Autodesk Inventor part; units mm, degrees
ref_plane "YZ Plane" through (0, 0, 0) normal (1, 0, 0) x (0, 1, 0)
ref_plane "XZ Plane" through (0, 0, 0) normal (0, 1, 0) x (-1, 0, 0)
ref_plane "XY Plane" through (0, 0, 0) normal (0, 0, 1) x (1, 0, 0)
sketch "Skizze5" plane through (0, 0, 0) normal (1, 0, 0) x (0, 1, 0)
  line L0 (0, 0) -> (0, 0)
  line L1 (0, 0) -> (4.4737, 0.486)
  line L2 (4.4737, 0.486) -> (10.9319, -0.2498)
  line L3 (10.9319, -0.2498) -> (10.9319, -0.2498)
  line L4 (10.9319, -0.2498) -> (10.9319, 5.2858)
  line L5 (10.9319, 5.2858) -> (4.4737, 6.0216)
  line L6 (0, 3.5206) -> (0, 0)
  line L7 (0, 3.5206) -> (4.4737, 4.0066)
  line L8 (4.4737, 8.0188) -> (4.4737, 2.9641) construction
  line L9 (4.4737, 6.0216) -> (4.4737, 4.0066)
  dimension "d21" = 0
  dimension "d22" = 6.2
  dimension "d23" = 6.5
  dimension "d24" = 4.5
  dimension "d25" = 6.5
  dimension "d26" = 5.5
  dimension "d27" = 3.5
extrude "Extrusion3" add sketch "Skizze5" along normal blind 8
sketch "Skizze6" plane through (8, 10.9319, -0.2498) normal (0, -0.1132, -0.9936) x (-1, 0, 0)
  circle A0 centre (4, -3.25) radius 2.425
  line L0 (4, 0.2781) -> (4, -10.3498)
  line L1 (-1.6335, -3.25) -> (9.1615, -3.25)
  line L2 (8, -6.5) -> (8, 0)
  line L3 (8, 0) -> (0, 0)
  point P0 (8, -10.8899)
  point P1 (8, -1.2477)
  point P2 (4, -0.9743)
  point P3 (8, -3.25)
  point P4 (4, 0)
  dimension "d30" = 4.85
extrude "Extrusion4" cut sketch "Skizze6" against normal through all contours L1 L0 A0 | A0 L0 L1 | L0 L1 A0 | A0 L1 L0
sketch "Skizze7" plane through (8, 4.4737, 0.486) normal (0, 0.108, -0.9942) x (-1, 0, 0)
  line L0 (-0.5646, -2.25) -> (9.8389, -2.25)
  line L1 (4, -0.832) -> (4, -8.1647)
  circle A0 centre (4, -2.25) radius 1.65
  line L2 (8, -4.5) -> (8, 0)
  line L3 (8, -4.5) -> (0, -4.5)
  point P0 (4, -5.6763)
  point P1 (8, -2.25)
  point P2 (8, -2.25)
  point P3 (4, -4.5)
  dimension "d33" = 3.3
extrude "Extrusion5" cut sketch "Skizze7" against normal through all contours A0 L0 | L0 L1 A0 | L0 A0 L1
chamfer "Fase2" distance 0.5 angle 45 4 edges at (8, 10.9319, 2.518) (0, 10.9319, 2.518) (8, 4.4737, 5.0141) (0, 4.4737, 5.0141)
ref_plane "Arbeitsebene3" through (0, 10.9319, -0.2498) normal (0, 0, 1) x (1, 0, 0)
sketch "Skizze11" plane through (0, 10.9319, -0.2498) normal (0, 0, 1) x (1, 0, 0)
  line L0 (0.5, 0) -> (7.5, 0)
  line L1 (8, -0.5) -> (7.5, 0)
  line L2 (8, -6.4582) -> (8, -0.5)
  line L3 (8, -10.9319) -> (8, -6.4582)
  line L4 (0, -10.9319) -> (8, -10.9319)
  line L5 (0, -10.9319) -> (0, -6.4582)
  line L6 (0, -6.4582) -> (0, -0.5)
  line L7 (0.5, 0) -> (0, -0.5)
extrude "Extrusion9" add sketch "Skizze11" along normal blind 1
sketch "Skizze12" plane through (0.5, 4.4737, 6.0216) normal (0, 0.1132, 0.9936) x (1, 0, 0)
  circle A0 centre (3.5, 3.8766) radius 2.425
  point P0 (-0.5, -3.7633)
extrude "Extrusion10" cut sketch "Skizze12" against normal through all
sketch "Skizze13" plane through (0, 0, 3.5206) normal (0, -0.108, 0.9942) x (1, 0, 0)
  circle A0 centre (4, 1.8698) radius 1.65
  point P0 (0, -0.3802)
extrude "Extrusion11" cut sketch "Skizze13" against normal through all
chamfer "Fase4" distance 0.5 angle 45 3 edges at (8, 5.2159, -0.2498) (4, 10.9319, -0.2498) (0, 5.2159, -0.2498)
chamfer "Fase5" distance 1.5 angle 45 2 edges at (8, 0, 1.8854) (0, 0, 1.8854)
properties part number "led_holder_v13"
Input: part model. Units: mm. Frame: model coordinates. A direction names the side the tool comes from. Coordinates: 2 decimals unless noted, no trailing zeros. Order: outer loops, then holes, each group sorted by start corner. A loop starts at its lowest first (then second) coordinate and runs counter-clockwise, first axis right, second up. Notation, with made-up numbers: M -11.5,74.25 L 39.5,74.25 A16 cw 39.5,97.25 Z; hole C 36.25,69.5 d5. An arc over 180 degrees is marked long. Answer in a Markdown table with one row per item.
(1) Material intervals for line 1 (Y direction, x = 3.5, z = 0.75); line 2 (Y direction, x = 3.75, z = 3); line 3 (Y direction, x = 1.25, z = 1.5), sorted ascending. Write a range as [from, to].
Numbers:
| item | result |
|---|---|
| line 1 | y = [0, 0.6], [3.76, 5.39], [10.16, 10.93] |
| line 2 | y = [0, 0.3], [3.58, 5.6], [10.46, 10.93] |
| line 3 | y = [0.25, 10.93] |
(2) Section query B-B, the plane x = 6.25. Output: boundary loops of the cut face in (y, z), plus the area to 3 significant figures.
Numbers:
| item | result |
|---|---|
| outline | M 0,-0.25 L 6.75,-0.25 L 7.43,5.69 L 4.47,6.02 L 4.47,4.01 L 0,3.52 Z; M 8.57,-0.25 L 10.43,-0.25 L 10.93,0.25 L 10.93,5.29 L 9.22,5.48 Z |
| area | 45.3 mm^2 |
(3) Contact query for flat-ended pins moving along their axis: pin 1 Ø0.6 at (x, z) = (2.5, 4.5) entering from -Y; pin 2 Ø4 at (x, y) = (5, 6.5) entering from -Z. Output: stop coordinate, or through.
Numbers:
| item | result |
|---|---|
| pin 1 | stops at y = 4.47 |
| pin 2 | stops at z = -0.25 |
(4) Section query D-D, the plane z = 1. Give the number of separate pieces and of enclosed holes in the cut face, plus the area to 3 significant figures.
Numbers:
| item | result |
|---|---|
| separate pieces | 1 |
| enclosed holes | 2 |
| area | 57.8 mm^2 |
(5) Access query for faces 1 (the flat face through (4, 0, 2)), 2 (the flat face through (4, 4.474, 5)). Directions: +Z, -Z, +X, -X, +Y, -Y. A direction counts if a zero-diameter tool reaches every point of the face in a straight line with its end or side. Return the directions, or none.
Numbers:
| item | result |
|---|---|
| face 1 | +Z, -Z, +X, -X, -Y |
| face 2 | +Z, +X, -X, -Y |
(6) Section query C-C, the plane x = 1. Output: boundary loops of the cut face in (y, z), plus the area to 3 significant figures.
Numbers:
| item | result |
|---|---|
| outline | M 0.5,-0.25 L 10.43,-0.25 L 10.93,0.25 L 10.93,5.29 L 4.47,6.02 L 4.47,4.01 L 0.5,3.57 Z |
| area | 54.1 mm^2 |
(7) Section query A-A, the plane x = 3. Output: boundary loops of the cut face in (y, z), plus the area to 3 significant figures.
Numbers:
| item | result |
|---|---|
| outline | M 0,-0.25 L 0.97,-0.25 L 0.55,3.58 L 0,3.52 Z; M 3.16,3.86 L 3.61,-0.25 L 5.44,-0.25 L 6.13,5.83 L 4.47,6.02 L 4.47,4.01 Z; M 9.88,-0.25 L 10.43,-0.25 L 10.93,0.25 L 10.93,5.29 L 10.52,5.33 Z |
| area | 19.5 mm^2 |
